from build123d import *

# Parameters (mm, degrees)
SKETCH_1_W      = 118
SKETCH_1_H      = 170
SKETCH_1_R      = 2
EXTRUDE_1_DEPTH = 3


with BuildPart() as part:
    # 草图1 → 凸台-拉伸1 (new body)
    with BuildSketch(Plane.XY):
        with Locations((0, 15)):
            Rectangle(SKETCH_1_W, SKETCH_1_H)
        with Locations((-49, 55)):
            Circle(SKETCH_1_R, mode=Mode.SUBTRACT)
        with Locations((-49, 45)):
            Circle(SKETCH_1_R, mode=Mode.SUBTRACT)
        with Locations(Location((49, 45, 0), (0, 0, 180))):
            Circle(SKETCH_1_R, mode=Mode.SUBTRACT)
        with Locations(Location((49, 55, 0), (0, 0, 180))):
            Circle(SKETCH_1_R, mode=Mode.SUBTRACT)
        with Locations((49, -45)):
            Circle(SKETCH_1_R, mode=Mode.SUBTRACT)
        with Locations((49, -55)):
            Circle(SKETCH_1_R, mode=Mode.SUBTRACT)
        with Locations(Location((-49, -45, 0), (0, 0, 180))):
            Circle(SKETCH_1_R, mode=Mode.SUBTRACT)
        with Locations(Location((-49, -55, 0), (0, 0, 180))):
            Circle(SKETCH_1_R, mode=Mode.SUBTRACT)
        with Locations((-47, 87.5)):
            Circle(SKETCH_1_R, mode=Mode.SUBTRACT)
        with Locations(Location((47, 87.5, 0), (0, 0, 180))):
            Circle(SKETCH_1_R, mode=Mode.SUBTRACT)
        with Locations((47, -31.5)):
            Circle(SKETCH_1_R, mode=Mode.SUBTRACT)
        with Locations(Location((-47, -31.5, 0), (0, 0, 180))):
            Circle(SKETCH_1_R, mode=Mode.SUBTRACT)
    extrude(amount=EXTRUDE_1_DEPTH)


solid = part.part
Geometry: final body of the model. Coordinates: model frame, mm. Coordinates: 2 decimals unless noted, no trailing zeros. Loops run counter-clockwise (first coordinate to the right, second up) from the corner with the lowest first, then second, coordinate; pieces in that order, holes last. Notation, with made-up numbers: M 89.25,36 L 143.25,36 A20 cw 143.25,49 Z; hole C -36.75,31.5 d6. An arc over 180 degrees is marked long. One line per item, written item: value. Start each with the question number.
1) Draft query along X for faces 1 (the flat face through (-1, 16, 0)), 2 (the cylindrical face through (49, -47, 1)). Return one class per face: released by +X, released by -X, zero draft, split by the parting line, or undercut.
2) Material intervals for L1, parallel to X at y = -33, z = 0.45, sorted ascending. Write a range as from..to.
3) Cut plane A-A (y = -31.5). Return loops of the section in (x, z), then the cut area to 3 significant figures.
Evaluation:
1. face 1: zero draft
1. face 2: undercut
2. L1: -59..-48.32, -45.68..45.68, 48.32..59
3. outline: M -59,0 L -49,0 L -49,3 L -59,3 Z; M -45,0 L 45,0 L 45,3 L -45,3 Z; M 49,0 L 59,0 L 59,3 L 49,3 Z
3. area: 330 mm^2
